```python
from build123d import *

# Parameters (mm, degrees)
F0_R     = 3.5
F1_DEPTH = 10
F2_R     = 2.6
F3_DEPTH = 4
F4_DEPTH = 7
F5_W     = 5
F5_H     = 1.5
F6_DEPTH = 6


with BuildPart() as f1:
    # F0 (on Top) → F1 (new body)
    with BuildSketch(Plane.XY):
        Circle(F0_R)
    extrude(amount=F1_DEPTH)

    # F2 (on face) → F3 (cut)
    with BuildSketch(Plane(origin=(0, 0, 0), x_dir=(1, 0, 0), z_dir=(0, 0, -1))):
        with Locations((0, 0.1646061121)):
            Circle(F2_R)
    extrude(amount=-F3_DEPTH, mode=Mode.SUBTRACT)

    # F4 (add): a face of the model
    f4_faces = [f1.faces().sort_by_distance(p)[0] for p in [
        (0, 0, 10),
    ]]
    extrude(f4_faces, amount=F4_DEPTH)

    # F5 (on face) → F6 (cut)
    with BuildSketch(Plane.XY.offset(17)):
        Rectangle(F5_W, F5_H)
    extrude(amount=-F6_DEPTH, mode=Mode.SUBTRACT)


solid = f1.part
```
Model file for the job. Use its own axes, mm. A direction names the side the tool comes from. Give positions to 0.01 mm unless a question says otherwise; leave off trailing zeros. Write each loop counter-clockwise with the first axis right and the second up, starting at its lowest first coordinate (ties: lowest second). Pieces come first, ordered by that corner, then holes. Notation, with made-up numbers: M 53.25,64.5 L 69.25,64.5 A32 cw 69.25,94.5 Z; hole C 48.25,17.25 d10. An arc over 180 degrees is marked long. Use a Markdown table: item, result.
1) Cut at A-A (z = 12.5). List the corners of the cut face in (x, y).
Responses:
| item | result |
|---|---|
| outline | C 0,0 d7; hole M -2.5,-0.75 L 2.5,-0.75 L 2.5,0.75 L -2.5,0.75 Z |
2) Tool access for faces 5 (the flat face through (2, 2, 0)), 6 (the flat face through (0, -0.75, 14)), 7 (the cylindrical face through (-0.338, -2.742, 1.972)): list every direction of +Z, -Z, +X, -X, +Y, -Y with a clear straight run to the whole face (end or side of a thin tool).
Responses:
| item | result |
|---|---|
| face 5 | -Z, +X, -X, +Y, -Y |
| face 6 | +Z |
| face 7 | -Z |
3) Cut at D-D (z = 5). List the corners of the cut face in (x, y), and give its area (3 significant figures).
Responses:
| item | result |
|---|---|
| outline | C 0,0 d7 |
| area | 38.5 mm2 |
4) Cut at B-B (x = 0). List the corners of the cut face in (y, z), and give its area (3 significant figures).
Responses:
| item | result |
|---|---|
| outline | M -3.5,0 L -2.76,0 L -2.76,4 L 2.44,4 L 2.44,0 L 3.5,0 L 3.5,17 L 0.75,17 L 0.75,11 L -0.75,11 L -0.75,17 L -3.5,17 Z |
| area | 89.2 mm2 |
5) Cut at C-C (y = -1.25). List the corners of the cut face in (x, z).
Responses:
| item | result |
|---|---|
| outline | M -3.27,0 L -2.36,0 L -2.36,4 L 2.36,4 L 2.36,0 L 3.27,0 L 3.27,17 L -3.27,17 Z |
6) Pin check, flat tips, straight feed: pin 1 (1.5 mm diameter, centred on y = -2, z = 7, fed in from -X); pin 2 (2 mm diameter, centred on y = 2, z = 7, fed in from +X); pin 3 (1.6 mm diameter, centred on x = 1, y = -1.5, fed in from -Z). Stop position of each tip, or through.
Responses:
| item | result |
|---|---|
| pin 1 | stops at x = -3.27 |
| pin 2 | stops at x = 3.35 |
| pin 3 | stops at z = 4 |
7) Drill centre lines: line 1 (Y direction, x = 0, z = 1.5); line 2 (Z direction, x = 2, y = 1); line 3 (Y direction, x = 0.25, z = 12.25). Where is each one in solid material? Low to high. Write a range as from..to.
Responses:
| item | result |
|---|---|
| line 1 | y = -3.5..-2.76, 2.44..3.5 |
| line 2 | z = 4..17 |
| line 3 | y = -3.49..-0.75, 0.75..3.49 |
8) Pull direction X, two halves, no side cores. Call faces 1 (the flat face through (2.5, 0, 14)), 2 (the flat face through (0, 1, 17)), 3 (the flat face through (0, 0, 11)), 4 (the cylindrical face through (3.233, -1.341, 8.381)): +X half, -X half, draft (parallel to the pull), parting line (faces both ways), or undercut.
Responses:
| item | result |
|---|---|
| face 1 | undercut |
| face 2 | draft |
| face 3 | undercut |
| face 4 | parting line |
